from build123d import *

# Parameters (mm, degrees)
F0_W      = 600
F0_H      = 2496
F1_DEPTH  = 1200
F2_W      = 1200
F2_H      = 96
F3_DEPTH  = 10
F4_W      = 1100
F4_H      = 160
F5_DEPTH  = 580
F7_W      = 1168
F7_H      = 2168
F8_DEPTH  = 586
F9_W      = 1168
F9_H      = 16
F10_DEPTH = 564
F11_W     = 16
F11_H     = 1768
F12_DEPTH = 564
F13_W     = 1168
F13_H     = 16
F14_DEPTH = 564


with BuildPart() as f1:
    # F0 (on Right) → F1 (new body)
    with BuildSketch(Plane.YZ):
        Rectangle(F0_W, F0_H)
    extrude(amount=F1_DEPTH)

    # F2 (on face) → F3 (cut)
    with BuildSketch(Plane.XZ.offset(300)):
        with Locations((600, -1200)):
            Rectangle(F2_W, F2_H)
    extrude(amount=-F3_DEPTH, mode=Mode.SUBTRACT)

    # F4 (on face) → F5 (cut)
    with BuildSketch(Plane.XZ.offset(300)):
        with Locations((600, -1052)):
            Rectangle(F4_W, F4_H)
    extrude(amount=-F5_DEPTH, mode=Mode.SUBTRACT)

    # F7 (on face) → F8 (cut)
    with BuildSketch(Plane.XZ.offset(300)):
        with Locations((600, 148)):
            Rectangle(F7_W, F7_H)
    extrude(amount=-F8_DEPTH, mode=Mode.SUBTRACT)

    # F9 (on offset) → F10 (join)
    with BuildSketch(Plane.XZ.offset(280)):
        with Locations((600, 840)):
            Rectangle(F9_W, F9_H)
    extrude(amount=-F10_DEPTH)

    # F11 (on offset) → F12 (join)
    with BuildSketch(Plane.XZ.offset(280)):
        with Locations((600, -52)):
            Rectangle(F11_W, F11_H)
    extrude(amount=-F12_DEPTH)

    # F13 (on offset) → F14 (join)
    with BuildSketch(Plane.XZ.offset(280)):
        with Locations((600, -678)):
            Rectangle(F13_W, F13_H)
        with Locations((600, -412)):
            Rectangle(F13_W, F13_H)
    extrude(amount=-F14_DEPTH)


solid = f1.part
Verification items for the finished model (mm, model axes). A direction names the side the tool comes from. Round coordinates to 2 decimals unless told otherwise and drop trailing zeros. Order: outer loops, then holes, each group sorted by start corner. A loop starts at its lowest first (then second) coordinate and runs counter-clockwise, first axis right, second up. Notation, with made-up numbers: (38, -40) -> (64, -40) arc R16 ccw to (64, -24) -> close; hole circle Ø2 at (34.25, -28). An arc over 180 degrees is marked (long way). Put each result on its own line as item: value.
1) Material ranges on line 1 (X direction, y = -211, z = -852.5); line 2 (Z direction, x = 656, y = 252); line 3 (X direction, y = 140.5, z = -1019.5), recorded low to high.
Final values:
line 1: x = 0 to 16, 592 to 608, 1184 to 1200
line 2: z = -1248 to -1132, -972 to -936, -686 to -670, -420 to -404, 832 to 848, 1232 to 1248
line 3: x = 0 to 50, 1150 to 1200
2) Section check B-B (z = 668). Record the cut outline in (x, y), then the cut area to 3 significant figures.
Final values:
outline: (0, -300) -> (16, -300) -> (16, 286) -> (1184, 286) -> (1184, -300) -> (1200, -300) -> (1200, 300) -> (0, 300) -> close; (592, -280) -> (608, -280) -> (608, 284) -> (592, 284) -> close
area: 44,600 mm^2
3) Set-up check for faces 4 (the flat face through (50, -14, -1053)), 5 (the flat face through (592, -290, -1199)), 6 (the flat face through (1200, -4, 17)): record each of +Z, -Z, +X, -X, +Y, -Y from which the full face is reachable in a straight line by a thin tool's end or side.
Final values:
face 4: -Y
face 5: -Z, +X, -X, -Y
face 6: +Z, -Z, +X, +Y, -Y
4) Section check A-A (x = 400). Record the cut outline in (y, z).
Final values:
outline: (-300, -1152) -> (-290, -1152) -> (-290, -1248) -> (300, -1248) -> (300, 1248) -> (-300, 1248) -> (-300, 1232) -> (286, 1232) -> (286, -936) -> (-300, -936) -> (-300, -972) -> (280, -972) -> (280, -1132) -> (-300, -1132) -> close; (-280, -686) -> (284, -686) -> (284, -670) -> (-280, -670) -> close; (-280, -420) -> (284, -420) -> (284, -404) -> (-280, -404) -> close; (-280, 832) -> (284, 832) -> (284, 848) -> (-280, 848) -> close
5) Mould release check, pull along Y, two halves, no side actions. Record for faces 1 (the flat face through (597, 284, -40)), 2 (the flat face through (592, 280, -1051)), 3 (the flat face through (591.8, -11.1, -936)): +Y half, -Y half, draft (parallel to the pull), parting line (faces both ways), or undercut.
Final values:
face 1: undercut
face 2: -Y half
face 3: draft
6) Depth check by flat-ended pin: pin 1 (1 mm diameter, centred on x = 424.5, z = -840.5, fed in from -Y). Enter the tip coordinate at first touch or a pass-through.
Final values:
pin 1: stops at y = 286
7) Section check C-C (y = -126). Give the number of separate pieces and of enclosed holes in the cut face, then the cut area to 3 significant figures.
Final values:
separate pieces: 1
enclosed holes: 8
area: 371,000 mm^2
